```python
from build123d import *

# Parameters (mm, degrees)
F0_R      = 26.67
F1_DEPTH  = 2
F5_DEPTH  = 8.42
F6_R      = 1.5
F8_DEPTH  = 8
F9_R      = 1.27
F11_DEPTH = 2
F10_R     = 2
F12_DEPTH = 1.3


with BuildPart() as f1:
    # F0 (on Top) → F1 (new body)
    with BuildSketch(Plane.XY):
        Circle(F0_R)
    extrude(amount=F1_DEPTH)

    # F4 (on face) → F5 (join)
    with BuildSketch(Plane.XY.offset(2)):
        with BuildLine():
            ThreePointArc((5.23, 26.15217), (0, 26.67), (-5.23, 26.15217))
            Line((-5.23, 26.15217), (-5.23, -26.15217))
            ThreePointArc((-5.23, -26.15217), (0, -26.67), (5.23, -26.15217))
            Line((5.23, -26.15217), (5.23, 26.15217))
        make_face()
    extrude(amount=F5_DEPTH)

    # F6
    f6_edges = [f1.edges().sort_by_distance(p)[0] for p in [
        (5.23, 0, 10.42),
        (0, 26.67, 10.42),
        (-5.23, 0, 10.42),
        (0, -26.67, 10.42),
    ]]
    fillet(f6_edges, radius=F6_R)

    # F7 (on face) → F8 (cut)
    with BuildSketch(Plane(origin=(0, 0, 0), x_dir=(1, 0, 0), z_dir=(0, 0, -1))):
        with BuildLine():
            ThreePointArc((3, 23.479116), (0, 23.67), (-3, 23.479116))
            Line((-3, 23.479116), (-3, -23.479116))
            ThreePointArc((-3, -23.479116), (0, -23.67), (3, -23.479116))
            Line((3, -23.479116), (3, 23.479116))
        make_face()
    extrude(amount=-F8_DEPTH, mode=Mode.SUBTRACT)

    # F9 (on face) → F11 (cut)
    with BuildSketch(Plane.XY.offset(2)):
        with Locations((-16.468517, 16.468517)):
            Circle(F9_R)
        with Locations((-16.468517, -16.468517)):
            Circle(F9_R)
        with Locations((16.468517, -16.468517)):
            Circle(F9_R)
        with Locations((16.468517, 16.468517)):
            Circle(F9_R)
    extrude(amount=-F11_DEPTH, mode=Mode.SUBTRACT)

    # F10 (on face) → F12 (cut)
    with BuildSketch(Plane.XY.offset(2)):
        with Locations((-16.468517, 16.468517)):
            Circle(F10_R)
        with Locations((-16.468517, -16.468517)):
            Circle(F10_R)
        with Locations((16.468517, -16.468517)):
            Circle(F10_R)
        with Locations((16.468517, 16.468517)):
            Circle(F10_R)
    extrude(amount=-F12_DEPTH, mode=Mode.SUBTRACT)


solid = f1.part
```
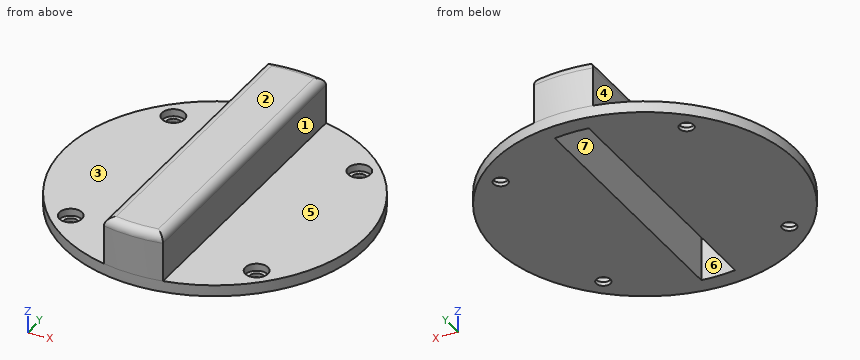
Could you check a few things on this model? Use its own coordinates, in mm. Face numbers are marked on the shaded views. A direction names the side the tool comes from. Round coordinates to 2 decimals unless told otherwise and drop trailing zeros. Loops run counter-clockwise (first coordinate to the right, second up) from the corner with the lowest first, then second, coordinate; pieces in that order, holes last. Notation, with made-up numbers: (-7, -11.5) -> (19, -11.5) arc R20 cw to (19, 24.5) -> close; hole circle Ø7 at (79.5, 64.5). An arc over 180 degrees is marked (long way). One line per question, with ' | ' between items.
(1) For pin 1 Ø2.5 at (y, z) = (7, 5.5) entering from +X; pin 2 Ø1.8 at (x, y) = (1, 3.5) entering from -Z; pin 3 Ø6.5 at (x, y) = (16.47, -16.47) entering from +Z, each with a flat end and sliding along its axis, tell me the tip position at first contact or that it passes through.
Model answer:
pin 1: stops at x = 5.23 | pin 2: stops at z = 8 | pin 3: stops at z = 2
(2) If we section it at D-D on x = 0: List the corners of the cut face in (y, z) for me, and give its area (3 significant figures).
Model answer:
outline: (-26.67, 0) -> (-23.67, 0) -> (-23.67, 8) -> (23.67, 8) -> (23.67, 0) -> (26.67, 0) -> (26.67, 8.92) arc R1.5 ccw to (25.17, 10.42) -> (-25.17, 10.42) arc R1.5 ccw to (-26.67, 8.92) -> close | area: 176 mm^2
(3) If we section it at A-A on z = 3: List the corners of the cut face in (x, y) for me.
Model answer:
outline: (-5.23, -26.15) arc R26.67 ccw to (5.23, -26.15) -> (5.23, 26.15) arc R26.67 ccw to (-5.23, 26.15) -> close; hole (-3, -23.48) arc R23.67 ccw to (3, -23.48) -> (3, 23.48) arc R23.67 ccw to (-3, 23.48) -> close
(4) If we section it at B-B on y = 0: List the corners of the cut face in (x, z) for me, and give its area (3 significant figures).
Model answer:
outline: (-26.67, 0) -> (-3, 0) -> (-3, 8) -> (3, 8) -> (3, 0) -> (26.67, 0) -> (26.67, 2) -> (5.23, 2) -> (5.23, 8.92) arc R1.5 ccw to (3.73, 10.42) -> (-3.73, 10.42) arc R1.5 ccw to (-5.23, 8.92) -> (-5.23, 2) -> (-26.67, 2) -> close | area: 146 mm^2
(5) For the marked faces 1, 2 and 3, which set-ups out of +Z, -Z, +X, -X, +Y, -Y let a thin tool reach every point of the face, with its end or its side?
Model answer:
face 1: +Z, +X, +Y, -Y | face 2: +Z, +X, -X, +Y, -Y | face 3: +Z, -X, +Y, -Y
(6) Thinking about a two-plate mould opening in X: for the marked faces 4, 5, 6 and 7, which applies, released by +X, released by -X, zero draft, split by the parting line, or undercut?
Model answer:
face 4: released by -X | face 5: zero draft | face 6: undercut | face 7: undercut
(7) If I drill on probe 1 along X at (y, z) = (10, 3); probe 2 along Z at (x, y) = (12.5, 0.5); probe 3 along X at (y, z) = (5, 8.75), over which ranges is the centre line in solid material (lowest first)?
Model answer:
probe 1: x = -5.23 to -3, 3 to 5.23 | probe 2: z = 0 to 2 | probe 3: x = -5.23 to 5.23
(8) If we section it at C-C on x = 16.5: List the corners of the cut face in (y, z) for me.
Model answer:
outline: (-20.95, 0) -> (-17.74, 0) -> (-17.74, 0.7) -> (-18.47, 0.7) -> (-18.47, 2) -> (-20.95, 2) -> close; (-15.2, 0) -> (15.2, 0) -> (15.2, 0.7) -> (14.47, 0.7) -> (14.47, 2) -> (-14.47, 2) -> (-14.47, 0.7) -> (-15.2, 0.7) -> close; (17.74, 0) -> (20.95, 0) -> (20.95, 2) -> (18.47, 2) -> (18.47, 0.7) -> (17.74, 0.7) -> close
